```python
from build123d import *

# Parameters (mm, degrees)
BASPROSKE_W        = 12
BASPROSKE_H        = 9
TOOTHCUT_DEPTH     = 18.492855685
TEETHCUTS_COUNT    = 18
TEETHCUTS_ANGLE    = 340
BORSKE_R           = 2
BORE_DEPTH         = 50.0000508
SKETCH2_R          = 3.25
CUT_EXTRUDE1_DEPTH = 3
SKETCH3_R          = 4.95
CUT_EXTRUDE2_DEPTH = 4


with BuildPart() as part:
    # BasProSke → Base-Revolve (revolve)
    with BuildSketch(Plane(origin=(0, 0, 0), x_dir=(1, 0, 0), z_dir=(0, 1, 0)), mode=Mode.PRIVATE) as base_revolve_sk:
        with Locations((6, 4.5)):
            Rectangle(BASPROSKE_W, BASPROSKE_H)
    revolve(base_revolve_sk.sketch.rotate(Axis((-10, 0, 0), (1, 0, 0)), 180), axis=Axis((-10, 0, 0), (1, 0, 0)))

    # TooCutSke → ToothCut (cut, through all)
    with BuildSketch(Plane(origin=(0, 0, 0), x_dir=(0, 0, -1), z_dir=(1, 0, 0))):
        with BuildLine():
            ThreePointArc((0.45926649, 6.958861278), (0, 6.974), (-0.45926649, 6.958861278))
            ThreePointArc((-0.45926649, 6.958861278), (-0.743858876, 8.01799277), (-1.365479267, 8.921508366))
            ThreePointArc((-1.365479267, 8.921508366), (0, 9.0254), (1.365479267, 8.921508366))
            ThreePointArc((1.365479267, 8.921508366), (0.743858876, 8.01799277), (0.45926649, 6.958861278))
        make_face()
    toothcut = extrude(amount=TOOTHCUT_DEPTH, mode=Mode.SUBTRACT)

    # TeethCuts: ToothCut ×18 about axis
    teethcuts_axis = Axis((-10, 0, 0), (1, 0, 0))
    for i in range(1, TEETHCUTS_COUNT):
        add(toothcut.rotate(teethcuts_axis, i * TEETHCUTS_ANGLE / (TEETHCUTS_COUNT - 1)), mode=Mode.SUBTRACT)

    # BorSke → Bore (cut, symmetric)
    with BuildSketch(Plane(origin=(0, 0, 0), x_dir=(0, 0, -1), z_dir=(1, 0, 0))):
        with Locations(Location((0, 0, 0), (0, 0, 180))):
            Circle(BORSKE_R)
    extrude(amount=BORE_DEPTH, both=True, mode=Mode.SUBTRACT)

    # Sketch2 → Cut-Extrude1 (cut)
    with BuildSketch(Plane(origin=(12, 0, 0), x_dir=(0, 0, -1), z_dir=(1, 0, 0))):
        Circle(SKETCH2_R)
    extrude(amount=-CUT_EXTRUDE1_DEPTH, mode=Mode.SUBTRACT)

    # Sketch3 → Cut-Extrude2 (cut)
    with BuildSketch(Plane.ZY):
        Circle(SKETCH3_R)
    extrude(amount=-CUT_EXTRUDE2_DEPTH, mode=Mode.SUBTRACT)


solid = part.part
```
Model file for the job. Use its own axes, mm. A direction names the side the tool comes from. Coordinates: 2 decimals unless noted, no trailing zeros. Write each loop counter-clockwise with the first axis right and the second up, starting at its lowest first coordinate (ties: lowest second). Pieces come first, ordered by that corner, then holes. Notation, with made-up numbers: (84.5, -39.5) - (127.5, -39.5) arc R20 cw to (127.5, -6.5) - close; hole circle Ø2 at (70, 83.5). An arc over 180 degrees is marked (long way). Use a Markdown table: item, result. Add a question column.
Item 1: Band-saw the part on A-A, the plane z = 0. Write the cut outline in (x, y), and give its area (3 significant figures).
Item 2: Drill centre lines: line 1 along Z through (x, y) = (8, 5.25); line 2 along X through (y, z) = (-4.5, 1.5); line 3 along Z through (x, y) = (5, -8). Where is each one in solid material? Low to high.
Item 3: Drop flat-ended pins along their axis: pin 1 (2 mm diameter, centred on x = 9, z = 0, fed in from -Y); pin 2 (2 mm diameter, centred on x = 7.5, y = 0.5, fed in from +Z); pin 3 (5 mm diameter, centred on y = 0, z = 0, fed in from +X); pin 4 (3.5 mm diameter, centred on y = 0, z = 0, fed in from +X). Give the stop position or say it passes through.
Item 4: 3-axis set-ups, long thin cutter, end or side, ignore diameter. For faces 1 (the face through (5.916, 5.664, -5.723)), 2 (the face through (4, -1, 2)), 3 (the face through (5.916, 2.107, -7.742)), 4 (the face through (5.916, -6.591, 4.576)): which of +Z, -Z, +X, -X, +Y, -Y reach the whole face in a straight line?
Item 5: Two-plate mould, pull along Z, no slides. Class faces 5 (the face through (5.92, -6.55, 2.39)), 6 (the face through (5.916, 4.628, -6.554)), 7 (the face through (5.916, 2.125, 7.767)): pulls with the +Z half, pulls with the -Z half, needs draft (parallel to the pull), parting line crosses it, or undercut.
Item 6: Band-saw the part on B-B, the plane y = -4.25. Write the cut outline in (x, z).
A:
| question | item | result |
|---|---|---|
| 1 | outline | (0, -6.97) - (12, -6.97) - (12, -3.25) - (9, -3.25) - (9, -2) - (4, -2) - (4, -4.95) - (0, -4.95) - close; (0, 4.95) - (4, 4.95) - (4, 2) - (9, 2) - (9, 3.25) - (12, 3.25) - (12, 6.97) - (0, 6.97) - close |
| 1 | area | 88.3 mm² |
| 2 | line 1 | z = -6.9 to -5.06, -4.59 to 4.59, 5.06 to 6.9 |
| 2 | line 2 | x = 4 to 12 |
| 2 | line 3 | z = -2.02 to -0.74, 0.74 to 2.02 |
| 3 | pin 1 | stops at y = -8.47 |
| 3 | pin 2 | stops at z = 9 |
| 3 | pin 3 | stops at x = 9 |
| 3 | pin 4 | passes through |
| 4 | face 1 | +X, -X, +Y |
| 4 | face 2 | -X |
| 4 | face 3 | -Z, +X, -X |
| 4 | face 4 | +X, -X |
| 5 | face 5 | undercut |
| 5 | face 6 | pulls with the -Z half |
| 5 | face 7 | pulls with the +Z half |
| 6 | outline | (0, -6.24) - (12, -6.24) - (12, 6.24) - (0, 6.24) - (0, 2.54) - (4, 2.54) - (4, -2.54) - (0, -2.54) - close |
